```python
from build123d import *

# Parameters (mm, degrees)
SKETCH1_R           = 8
SKETCH1_R_2         = 4
BOSS_EXTRUDE1_DEPTH = 2


with BuildPart() as part:
    # Sketch1 → Boss-Extrude1 (new body, symmetric)
    with BuildSketch(Plane(origin=(0, 0, 0), x_dir=(1, 0, 0), z_dir=(0, 1, 0))):
        with BuildLine():
            Line((-61, 12.5), (61, 12.5))
            ThreePointArc((61, 12.5), (73.5, 0), (61, -12.5))
            Line((61, -12.5), (-61, -12.5))
            ThreePointArc((-61, -12.5), (-73.5, 0), (-61, 12.5))
        make_face()
        with Locations((-61, 0)):
            Circle(SKETCH1_R, mode=Mode.SUBTRACT)
        with Locations((1, 0)):
            Circle(SKETCH1_R_2, mode=Mode.SUBTRACT)
        with Locations((16, 0)):
            Circle(SKETCH1_R_2, mode=Mode.SUBTRACT)
        with Locations((31, 0)):
            Circle(SKETCH1_R_2, mode=Mode.SUBTRACT)
        with Locations((46, 0)):
            Circle(SKETCH1_R_2, mode=Mode.SUBTRACT)
        with Locations((61, 0)):
            Circle(SKETCH1_R_2, mode=Mode.SUBTRACT)
    extrude(amount=BOSS_EXTRUDE1_DEPTH, both=True)


solid = part.part
```
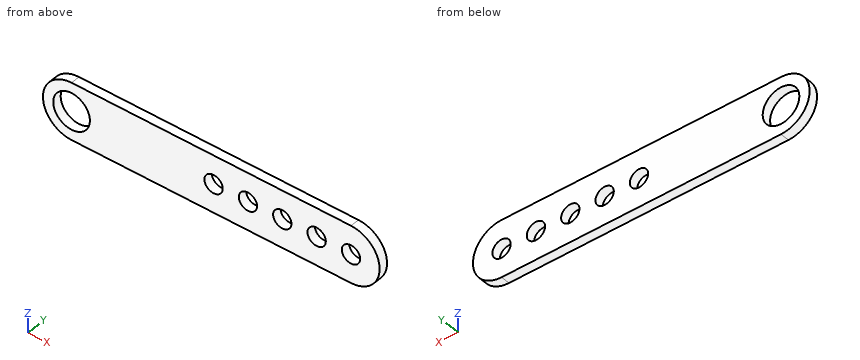
Model file for the job. Use its own axes, mm. Give positions to 0.01 mm unless a question says otherwise; leave off trailing zeros. Loops run counter-clockwise (first coordinate to the right, second up) from the corner with the lowest first, then second, coordinate; pieces in that order, holes last. Notation, with made-up numbers: (4.25, 39) -> (29.25, 39) arc R24 cw to (29.25, 71) -> close; hole circle Ø10 at (14.25, 44.25). An arc over 180 degrees is marked (long way). Use CSV: the item, a comma, the result in double quotes. Start each with the question number.
1) Slice it at D-D on z = 5.5. Give the cut face in (x, y).
2) Wall check: line 1 (Z direction, x = -61, y = 1.05); line 2 (Z direction, x = 1, y = -0.6); line 3 (X direction, y = 1.6, z = -5.75). Give the ranges that are in metal, low to high.
3) Slice it at C-C on x = 31. Give the cut face in (y, z).
4) Slice it at A-A on z = 0. Give the cut face in (x, y).
5) Slice it at B-B on y = -1.3. Give the cut face in (x, z).
Computed values:
1,outline,"(-72.22, -2) -> (-66.81, -2) -> (-66.81, 2) -> (-72.22, 2) -> close; (-55.19, -2) -> (72.22, -2) -> (72.22, 2) -> (-55.19, 2) -> close"
2,line 1,"z = -12.5 to -8, 8 to 12.5"
2,line 2,"z = -12.5 to -4, 4 to 12.5"
2,line 3,"x = -72.1 to -66.56, -55.44 to 72.1"
3,outline,"(-2, -12.5) -> (2, -12.5) -> (2, -4) -> (-2, -4) -> close; (-2, 4) -> (2, 4) -> (2, 12.5) -> (-2, 12.5) -> close"
4,outline,"(-73.5, -2) -> (-69, -2) -> (-69, 2) -> (-73.5, 2) -> close; (-53, -2) -> (-3, -2) -> (-3, 2) -> (-53, 2) -> close; (5, -2) -> (12, -2) -> (12, 2) -> (5, 2) -> close; (20, -2) -> (27, -2) -> (27, 2) -> (20, 2) -> close; (35, -2) -> (42, -2) -> (42, 2) -> (35, 2) -> close; (50, -2) -> (57, -2) -> (57, 2) -> (50, 2) -> close; (65, -2) -> (73.5, -2) -> (73.5, 2) -> (65, 2) -> close"
5,outline,"(-61, -12.5) -> (61, -12.5) arc R12.5 ccw to (61, 12.5) -> (-61, 12.5) arc R12.5 ccw to start; hole circle Ø16 at (-61, 0); hole circle Ø8 at (1, 0); hole circle Ø8 at (16, 0); hole circle Ø8 at (31, 0); hole circle Ø8 at (46, 0); hole circle Ø8 at (61, 0)"
